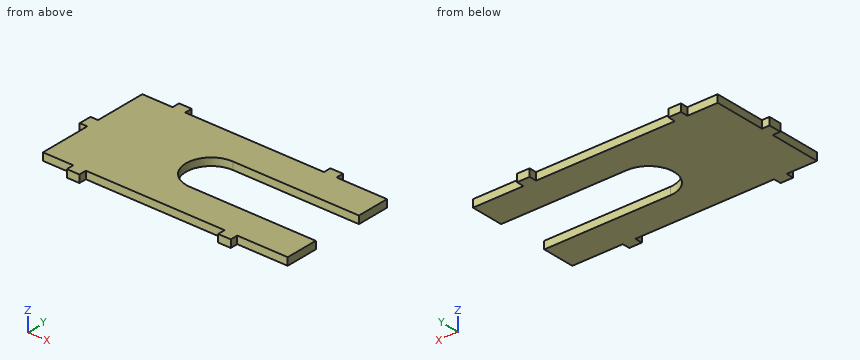
from build123d import *

# Parameters (mm, degrees)
F0_W     = 100
F0_H     = 52
F1_DEPTH = 3
F3_W     = 12
F3_H     = 3
F3_W_2   = 3
F3_H_2   = 20.5
F3_W_3   = 55
F3_W_4   = 17
F4_DEPTH = 3.001
F6_DEPTH = 3.001


with BuildPart() as f1:
    # F0 (on Top) → F1 (new body)
    with BuildSketch(Plane.XY):
        Rectangle(F0_W, F0_H)
    extrude(amount=F1_DEPTH)

    # F3 (on face) → F4 (cut, through all)
    with BuildSketch(Plane.XY.offset(3)):
        with Locations((-41, 24.5)):
            Rectangle(F3_W, F3_H)
        with Locations((-48.5, 24.5)):
            Rectangle(F3_W_2, F3_H)
        with Locations((-48.5, 12.75)):
            Rectangle(F3_W_2, F3_H_2)
        with Locations((-48.5, -12.75)):
            Rectangle(F3_W_2, F3_H_2)
        with Locations((-48.5, -24.5)):
            Rectangle(F3_W_2, F3_H)
        with Locations((-41, -24.5)):
            Rectangle(F3_W, F3_H)
        with Locations((-2.5, -24.5)):
            Rectangle(F3_W_3, F3_H)
        with Locations((38.5, -24.5)):
            Rectangle(F3_W_4, F3_H)
        with Locations((48.5, -24.5)):
            Rectangle(F3_W_2, F3_H)
        with Locations((48.5, 24.5)):
            Rectangle(F3_W_2, F3_H)
        with Locations((38.5, 24.5)):
            Rectangle(F3_W_4, F3_H)
        with Locations((-2.5, 24.5)):
            Rectangle(F3_W_3, F3_H)
    extrude(amount=-F4_DEPTH, mode=Mode.SUBTRACT)

    # F5 (on face) → F6 (cut, through all)
    with BuildSketch(Plane.XY.offset(3)):
        with BuildLine():
            ThreePointArc((0, -10), (7.071068, -7.071068), (10, 0))
            ThreePointArc((10, 0), (7.071068, 7.071068), (0, 10))
            ThreePointArc((0, 10), (-10, 0), (0, -10))
        make_face()
        with BuildLine():
            ThreePointArc((0, 10), (7.071068, 7.071068), (10, 0))
            ThreePointArc((10, 0), (7.071068, -7.071068), (0, -10))
            Line((0, -10), (50, -10))
            Line((50, -10), (50, 10))
            Line((50, 10), (0, 10))
        make_face()
    extrude(amount=-F6_DEPTH, mode=Mode.SUBTRACT)


solid = f1.part
For this review, take the finished solid that the model builds, in its own axes (mm). Coordinates: 2 decimals unless noted, no trailing zeros. Loops run counter-clockwise (first coordinate to the right, second up) from the corner with the lowest first, then second, coordinate; pieces in that order, holes last. Notation, with made-up numbers: (9, 62) - (39, 62) arc R24 ccw to (39, 80) - close; hole circle Ø5 at (61.5, -37.5). An arc over 180 degrees is marked (long way). Return JSON: item names as keys, results as strings.
Item 1: Take a section at C-C (x = -20.5). Give the boundary of the cut face in (y, z).
Determined:
{"outline": "(-23, 0) - (23, 0) - (23, 3) - (-23, 3) - close"}
Item 2: Take a section at D-D (y = 20). Give the boundary of the cut face in (x, z).
Determined:
{"outline": "(-47, 0) - (50, 0) - (50, 3) - (-47, 3) - close"}
Item 3: Take a section at A-A (x = 43.5). Give the boundary of the cut face in (y, z), then the cut area to 3 significant figures.
Determined:
{"outline": "(-23, 0) - (-10, 0) - (-10, 3) - (-23, 3) - close; (10, 0) - (23, 0) - (23, 3) - (10, 3) - close", "area": "78.0 mm2"}
Item 4: Take a section at B-B (z = 2.5). Give the boundary of the cut face in (x, y).
Determined:
{"outline": "(-50, -2.5) - (-47, -2.5) - (-47, -23) - (-35, -23) - (-35, -26) - (-30, -26) - (-30, -23) - (25, -23) - (25, -26) - (30, -26) - (30, -23) - (50, -23) - (50, -10) - (0, -10) arc R10 cw to (0, 10) - (50, 10) - (50, 23) - (30, 23) - (30, 26) - (25, 26) - (25, 23) - (-30, 23) - (-30, 26) - (-35, 26) - (-35, 23) - (-47, 23) - (-47, 2.5) - (-50, 2.5) - close"}
Item 5: Insertion check: pin 1 (1.5 mm diameter, centred on x = 36.5, z = 1, fed in from -Y); pin 2 (1 mm diameter, centred on y = -5.5, z = 2, fed in from +X); pin 3 (1.5 mm diameter, centred on x = -48.5, z = 2, fed in from -Y). Each pin has a flat end and moves straight along its axis. Give the tip position at first contact, or say it passes through.
Determined:
{"pin 1": "stops at y = -23", "pin 2": "stops at x = -8", "pin 3": "stops at y = -2.5"}
Item 6: For line 1 (Y direction, x = 20, z = 1.05); line 2 (X direction, y = 21, z = 2.15); line 3 (Y direction, x = -27, z = 0.5), list the stretches that pass through material, from the lowest coordinate up.
Determined:
{"line 1": "y = -23 to -10, 10 to 23", "line 2": "x = -47 to 50", "line 3": "y = -23 to 23"}
